Model file for the job. Use its own axes, mm. Coordinates: 2 decimals unless noted, no trailing zeros. Order: outer loops, then holes, each group sorted by start corner. A loop starts at its lowest first (then second) coordinate and runs counter-clockwise, first axis right, second up. Notation, with made-up numbers: (13.25, 53) - (19.25, 53) arc R16 ccw to (19.25, 77) - close; hole circle Ø7 at (-19, 67.5). An arc over 180 degrees is marked (long way). Put each result on its own line as item: value. Start each with the question number.
```python
from build123d import *

# Parameters (mm, degrees)
PAD_DEPTH = 20
FILLET_R  = 2


with BuildPart() as part:
    # Sketch → Pad (new body)
    with BuildSketch(Plane.XZ):
        Polygon((0, 0), (0, 22), (80, 10), (80, 0), align=None)
    extrude(amount=PAD_DEPTH)

    # Fillet
    fillet_edges = [part.edges().sort_by_distance(p)[0] for p in [
        (0, -10, 0),
        (0, -10, 22),
        (0, 0, 11),
        (0, -20, 11),
        (80, -10, 10),
        (40, 0, 16),
        (40, -20, 16),
        (80, -10, 0),
        (80, 0, 5),
        (80, -20, 5),
        (40, 0, 0),
        (40, -20, 0),
    ]]
    fillet(fillet_edges, radius=FILLET_R)


solid = part.part
```
Item 1: Slice it at A-A, the plane y = -13.5. Give the cut face in (x, z), plus the area to 3 significant figures.
Item 2: Flat gauge pins, fed straight in: pin 1 Ø4 at (x, z) = (44.5, 19) entering from +Y; pin 2 Ø10 at (x, y) = (13, -9) entering from +Z; pin 3 Ø5 at (x, y) = (49.5, -14) entering from +Z. Where does each tip first touch, or does it go through?
Item 3: Wall check: line 1 along X through (y, z) = (-17, 8.5); line 2 along Z through (x, y) = (73, -6.25); line 3 along X through (y, z) = (-2.25, 9). Give the ranges that are in metal, low to high.
Here are the results:
1. outline: (0, 2) arc R2 ccw to (2, 0) - (78, 0) arc R2 ccw to (80, 2) - (80, 8.28) arc R2 ccw to (78.3, 10.26) - (2.3, 21.66) arc R2 ccw to (0, 19.68) - close
1. area: 1,280 mm^2
2. pin 1: passes through
2. pin 2: stops at z = 20.8
2. pin 3: stops at z = 14.95
3. line 1: x = 0 to 79.99
3. line 2: z = 0 to 11.05
3. line 3: x = 0 to 79.86
